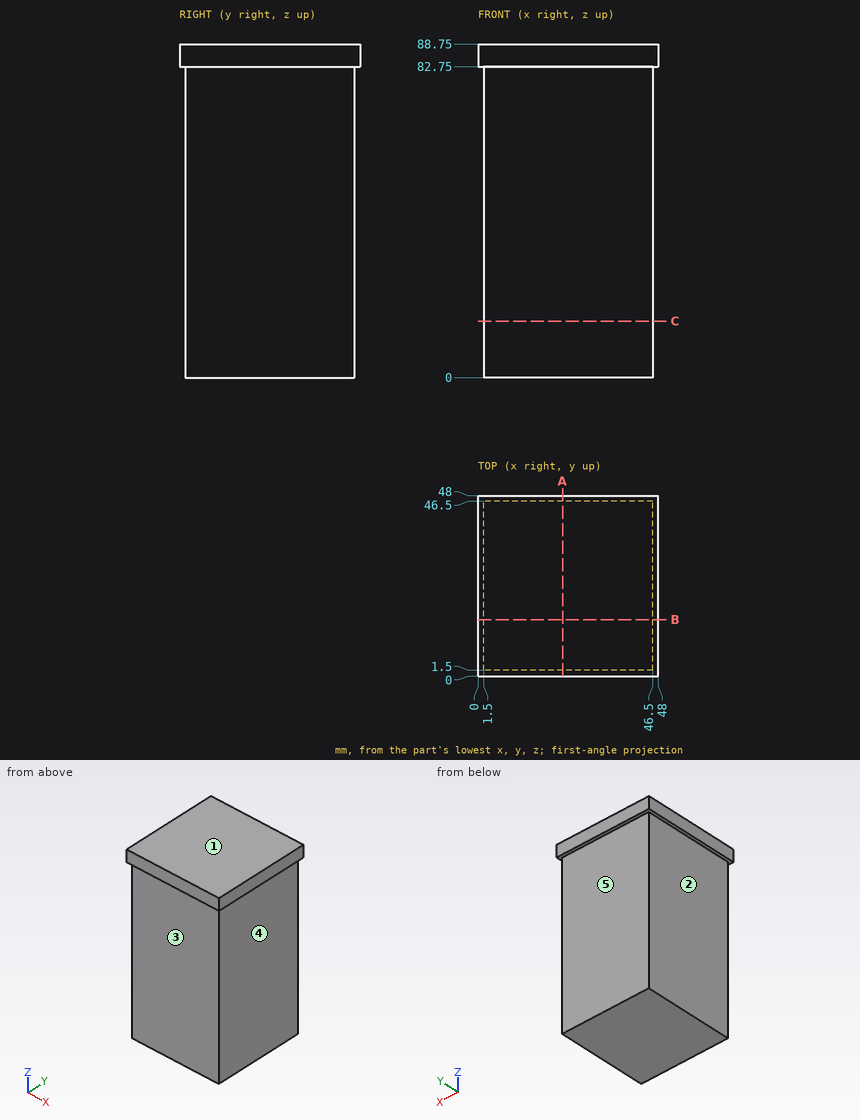
The figure shows three views and two pictorial views of one solid part (mm, origin at its lowest corner). Answer the questions. A direction names the side the tool comes from. Give positions to 0.01 mm unless a question says otherwise; leave off trailing zeros. Write each loop counter-clockwise with the first axis right and the second up, starting at its lowest first coordinate (ties: lowest second). Pieces come first, ordered by that corner, then holes. Notation, with made-up numbers: M -16,33 L 1,33 A14 cw 1,43 Z; hole C -36.75,-27.5 d9. An arc over 180 degrees is marked long. One line per item, written item: value. Start each with the question number.
(1) A tool of negligible diameter and unlimited length cuts with its end or side. For the marked faces 1, 2, 3, 4 and 5, from which of +Z, -Z, +X, -X, +Y, -Y can it reach the whole face along a straight path? Write none if from no direction.
(2) Find the intervals of material crossed by line 1 (X direction, y = 34.5, z = 6.5), in increasing order.
(3) Find section A-A (x = 22.5). Determine the outline of the cut face in (y, z).
(4) Flat-ended cylindrical pins translate along their axes: pin 1 Ø4 at (x, y) = (37.5, 18) entering from -Z; pin 2 Ø3 at (x, z) = (11, 42.5) entering from +Y; pin 3 Ø3 at (y, z) = (24.5, 61.5) entering from -X; pin 4 Ø1 at (x, z) = (8.5, 18) entering from -Y. Find the tip coordinate at first contact, or state that the pin passes through.
(5) Find section C-C (z = 15). Determine the outline of the cut face in (x, y), plus the area to 4 significant figures.
Results below:
1. face 1: +Z, +X, -X, +Y, -Y
1. face 2: -Z, -X, +Y, -Y
1. face 3: -Z, +X, -X, -Y
1. face 4: -Z, +X, +Y, -Y
1. face 5: -Z, +X, -X, +Y
2. line 1: x = 1.5 to 46.5
3. outline: M 0,82.75 L 1.5,82.75 L 1.5,0 L 46.5,0 L 46.5,82.75 L 48,82.75 L 48,88.75 L 0,88.75 Z
4. pin 1: stops at z = 0
4. pin 2: stops at y = 46.5
4. pin 3: stops at x = 1.5
4. pin 4: stops at y = 1.5
5. outline: M 1.5,1.5 L 46.5,1.5 L 46.5,46.5 L 1.5,46.5 Z
5. area: 2,025 mm^2
